```python
from build123d import *

# Parameters (mm, degrees)
P_IDAT_VYSUNUT_M1_DEPTH  = 8
SKICA2_R                 = 2.2
ODEBRAT_VYSUNUT_M1_DEPTH = 8
P_IDAT_VYSUNUT_M3_DEPTH  = 15
ZAOBLIT3_R               = 10
ZAOBLIT5_R               = 2
ZAOBLIT6_R               = 2
ZAOBLIT7_R               = 2
P_IDAT_VYSUNUT_M6_DEPTH  = 23
ZAOBLIT12_R              = 2
ZAOBLIT13_R              = 2
ZAOBLIT14_R              = 2
ZAOBLIT15_R              = 2
ODEBRAT_VYSUNUT_M4_DEPTH = 8.5
ZAOBLIT18_R              = 2
ZAOBLIT19_R              = 2
SKICA8_R                 = 0.5000000000000009
SKICA8_W                 = 12.000000000000004
SKICA8_H                 = 9
ODEBRAT_VYSUNUT_M5_DEPTH = 2
SKICA9_W                 = 12.000000000000004
SKICA9_H                 = 9
ODEBRAT_VYSUNUT_M6_DEPTH = 2.5


with BuildPart() as part:
    # Skica1 → Přidat vysunutím1 (new body)
    with BuildSketch(Plane.XY):
        Polygon((0, 0), (0, 25), (35, 25.000000000000004), (35, -3.47e-15), align=None)
        Polygon((3.999999999999999, 18.500000000000004), (4, 6.500000000000001), (18, 6.500000000000001), (20.485281374238575, 12.499999999999996), (18, 18.499999999999996), align=None, mode=Mode.SUBTRACT)
    extrude(amount=P_IDAT_VYSUNUT_M1_DEPTH)

    # Skica2 → Odebrat vysunutím1 (cut)
    with BuildSketch(Plane.ZY):
        with Locations((4, 12.5)):
            Circle(SKICA2_R)
    extrude(amount=-ODEBRAT_VYSUNUT_M1_DEPTH, mode=Mode.SUBTRACT)

    # Skica3 → Přidat vysunutím3 (add)
    with BuildSketch(Plane(origin=(0, 0, 0), x_dir=(-1, 0, 0), z_dir=(0, 0, -1))):
        Polygon((-35, 25.000000000000004), (-22, 25.000000000000004), (-21.999999999999996, 0), (-35, 0), align=None)
    extrude(amount=P_IDAT_VYSUNUT_M3_DEPTH)

    # Zaoblit3
    # the kernel refuses this fillet: 10 mm, written as the material it adds along each edge
    with BuildSketch(Plane(origin=(22, 25.000000000000004, 0), x_dir=(0, 0, -1), z_dir=(-1.4e-16, -1, 0))) as zaoblit3_piece_1_section:
        with BuildLine():
            CenterArc((ZAOBLIT3_R, -ZAOBLIT3_R), ZAOBLIT3_R, 90, 90)
            Line((-1.78e-15, -ZAOBLIT3_R), (0, 0))
            Line((0, 0), (ZAOBLIT3_R, 0))
        make_face()
    zaoblit3_piece_1 = extrude(amount=49.99999999999999, mode=Mode.PRIVATE)
    zaoblit3_piece_1 = split(zaoblit3_piece_1, bisect_by=Plane(origin=(17.13517134220591, 20.587881074775396, -2.4104777479798574), z_dir=(0.9238795325112865, 0.3826834323650904, 0)), keep=Keep.TOP, mode=Mode.PRIVATE)
    add(zaoblit3_piece_1)
    with BuildSketch(Plane(origin=(22, 25.000000000000004, 0), x_dir=(0, 0, -1), z_dir=(-1.4e-16, -1, 0))) as zaoblit3_piece_2_section:
        with BuildLine():
            CenterArc((ZAOBLIT3_R, -ZAOBLIT3_R), ZAOBLIT3_R, 90, 90)
            Line((-1.78e-15, -ZAOBLIT3_R), (0, 0))
            Line((0, 0), (ZAOBLIT3_R, 0))
        make_face()
    zaoblit3_piece_2 = extrude(amount=49.99999999999999, mode=Mode.PRIVATE)
    zaoblit3_piece_2 = split(zaoblit3_piece_2, bisect_by=Plane(origin=(15.789776111016284, 18.499999999999996, -0.41218867261979963), z_dir=(5.1e-16, 1, 0)), keep=Keep.TOP, mode=Mode.PRIVATE)
    add(zaoblit3_piece_2)
    with BuildSketch(Plane(origin=(22.000000000000004, 50, 0), x_dir=(0, 0, -1), z_dir=(-1.4e-16, -1, 0))) as zaoblit3_piece_3_section:
        with BuildLine():
            CenterArc((ZAOBLIT3_R, -ZAOBLIT3_R), ZAOBLIT3_R, 90, 90)
            Line((-1.78e-15, -ZAOBLIT3_R), (0, 0))
            Line((0, 0), (ZAOBLIT3_R, 0))
        make_face()
    zaoblit3_piece_3 = extrude(amount=50, mode=Mode.PRIVATE)
    zaoblit3_piece_3 = split(zaoblit3_piece_3, bisect_by=Plane(origin=(15.78977611101612, 6.500000000000001, -0.41218867261958336), z_dir=(0, -1, 0)), keep=Keep.TOP, mode=Mode.PRIVATE)
    add(zaoblit3_piece_3)
    with BuildSketch(Plane(origin=(22.000000000000004, 50, 0), x_dir=(0, 0, -1), z_dir=(-1.4e-16, -1, 0))) as zaoblit3_piece_4_section:
        with BuildLine():
            CenterArc((ZAOBLIT3_R, -ZAOBLIT3_R), ZAOBLIT3_R, 90, 90)
            Line((-1.78e-15, -ZAOBLIT3_R), (0, 0))
            Line((0, 0), (ZAOBLIT3_R, 0))
        make_face()
    zaoblit3_piece_4 = extrude(amount=50, mode=Mode.PRIVATE)
    zaoblit3_piece_4 = split(zaoblit3_piece_4, bisect_by=Plane(origin=(19.135383660262896, 9.241058631103481, -2.632109872171155), z_dir=(0.9238795325112864, -0.38268343236509067, 0)), keep=Keep.TOP, mode=Mode.PRIVATE)
    add(zaoblit3_piece_4)

    # Zaoblit5
    # the kernel refuses this fillet: 2 mm, written as the material it takes off along each edge
    with BuildSketch(Plane(origin=(0, -5, 0), x_dir=(0, 0, 1), z_dir=(0, 1, 0))) as zaoblit5_piece_1:
        with BuildLine():
            CenterArc((ZAOBLIT5_R, ZAOBLIT5_R), ZAOBLIT5_R, 180, 90)
            Line((-2.2e-16, ZAOBLIT5_R), (0, 0))
            Line((0, 0), (ZAOBLIT5_R, 0))
        make_face()
    extrude(amount=35, mode=Mode.SUBTRACT)

    # Zaoblit6
    zaoblit6_edges = [part.edges().sort_by_distance(p)[0] for p in [
        (21.999999999999996, 0, -12.5),
        (19.071067811865476, 0, -2.9289321881345254),
        (7, -6.9e-16, 0),
        (0.5857864376269049, 0, 0.5857864376269051),
        (0, 0, 5),
    ]]
    fillet(zaoblit6_edges, radius=ZAOBLIT6_R)

    # Zaoblit7
    zaoblit7_edges = [part.edges().sort_by_distance(p)[0] for p in [
        (22, 25.000000000000004, -12.5),
        (7, 25, 0),
        (19.071067811865476, 25, -2.9289321881345245),
        (0.5857864376269049, 25, 0.5857864376269051),
        (0, 25, 5),
    ]]
    fillet(zaoblit7_edges, radius=ZAOBLIT7_R)

    # Skica6 → Přidat vysunutím6 (add)
    with BuildSketch(Plane(origin=(0, 0, -15), x_dir=(-1, 0, 0), z_dir=(0, 0, -1))):
        with BuildLine():
            Line((-35, 23.500000000000004), (-35, 1.5))
            ThreePointArc((-35, 1.5), (-35.60000000229765, 2.1000000000000085), (-36.2, 1.4999999954047263))
            ThreePointArc((-36.2, 1.4999999954047263), (-36.58, 1.1199999924943909), (-36.96, 1.4999999954047263))
            Line((-36.96, 1.4999999954047263), (-36.959999999999994, 23.500000000000096))
            ThreePointArc((-36.959999999999994, 23.500000000000096), (-36.58, 23.88000000000009), (-36.2, 23.500000000000096))
            ThreePointArc((-36.2, 23.500000000000096), (-35.60000000000006, 22.9), (-35, 23.500000000000004))
        make_face()
    extrude(amount=-P_IDAT_VYSUNUT_M6_DEPTH)

    # Zaoblit12
    zaoblit12_edges = [part.edges().sort_by_distance(p)[0] for p in [
        (29.5, 0, -15),
        (22.5857864376269, 0.5857864376269046, -15),
        (29.5, 25.000000000000004, -15),
        (22.585786437626904, 24.414213562373096, -15),
        (21.999999999999996, 12.5, -15),
    ]]
    fillet(zaoblit12_edges, radius=ZAOBLIT12_R)

    # Zaoblit13
    zaoblit13_edges = [part.edges().sort_by_distance(p)[0] for p in [
        (20.485281374238724, 12.499999999999886, 1.6457513110643447),
    ]]
    fillet(zaoblit13_edges, radius=ZAOBLIT13_R)

    # Zaoblit14
    zaoblit14_edges = [part.edges().sort_by_distance(p)[0] for p in [
        (17.99999999999998, 18.500000000000004, 3.000000000000016),
    ]]
    fillet(zaoblit14_edges, radius=ZAOBLIT14_R)

    # Zaoblit15
    zaoblit15_edges = [part.edges().sort_by_distance(p)[0] for p in [
        (18.0000000000001, 6.499999999999996, 2.9999999999999263),
    ]]
    fillet(zaoblit15_edges, radius=ZAOBLIT15_R)

    # Skica7 → Odebrat vysunutím4 (cut)
    with BuildSketch(Plane(origin=(36.96, 1.166e-14, 0), x_dir=(0, 0, -1), z_dir=(1, 0, 0))):
        Polygon((-8, 21.00000000000012), (15, 21.00000000000012), (15.000000000000005, 4.000000000000118), (-7.999999999999998, 4.000000000000118), align=None)
    extrude(amount=-ODEBRAT_VYSUNUT_M4_DEPTH, mode=Mode.SUBTRACT)

    # Zaoblit18
    zaoblit18_edges = [part.edges().sort_by_distance(p)[0] for p in [
        (36.96, 21.00000000000013, -3.5),
    ]]
    fillet(zaoblit18_edges, radius=ZAOBLIT18_R)

    # Zaoblit19
    zaoblit19_edges = [part.edges().sort_by_distance(p)[0] for p in [
        (36.96, 4.00000000000013, -3.5000000000000036),
    ]]
    fillet(zaoblit19_edges, radius=ZAOBLIT19_R)

    # Skica8 → Odebrat vysunutím5 (cut)
    with BuildSketch(Plane(origin=(28.46, 0, 0), x_dir=(0, 0, -1), z_dir=(1, 0, 0))):
        with Locations((-4.750000000000001, 18.50000000000013)):
            Circle(SKICA8_R)
        with Locations((-4.750000000000001, 6.500000000000129)):
            Circle(SKICA8_R)
        with Locations((10.750000000000002, 18.50000000000013)):
            Circle(SKICA8_R)
        with Locations((10.750000000000002, 6.500000000000129)):
            Circle(SKICA8_R)
        with Locations((3.000000000000002, 12.500000000000128)):
            Rectangle(SKICA8_W, SKICA8_H)
    extrude(amount=-ODEBRAT_VYSUNUT_M5_DEPTH, mode=Mode.SUBTRACT)

    # Skica9 → Odebrat vysunutím6 (cut)
    with BuildSketch(Plane(origin=(28.46, 0, 0), x_dir=(0, 0, -1), z_dir=(1, 0, 0))):
        Polygon((-3.250000000000001, 17.000000000000128), (-5.999999999999998, 17.000000000000128), (-5.999999999999997, 8.000000000000128), (-3.2500000000000004, 8.000000000000128), (-2.9999999999999987, 8.000000000000128), (-2.9999999999999987, 17.000000000000128), align=None)
        Polygon((-3.250000000000001, 18.50000000000013), (-3.250000000000001, 17.000000000000128), (-2.9999999999999987, 17.000000000000128), (9.000000000000004, 17.000000000000128), (9.250000000000002, 17.000000000000128), (9.250000000000002, 18.50000000000013), align=None)
        Polygon((9.250000000000002, 17.000000000000128), (9.000000000000004, 17.000000000000128), (9.000000000000004, 8.000000000000128), (9.250000000000004, 8.000000000000128), (13.500000000000004, 8.000000000000128), (13.500000000000002, 17.000000000000128), align=None)
        with Locations((3.000000000000002, 12.500000000000128)):
            Rectangle(SKICA9_W, SKICA9_H)
        Polygon((-2.9999999999999987, 8.000000000000128), (-3.2500000000000004, 8.000000000000128), (-3.2500000000000004, 6.500000000000129), (9.250000000000002, 6.500000000000129), (9.250000000000002, 8.000000000000128), (9.000000000000004, 8.000000000000128), align=None)
    extrude(amount=-ODEBRAT_VYSUNUT_M6_DEPTH, mode=Mode.SUBTRACT)


solid = part.part
```
Here's how the part is built. I have some questions about the finished solid (model axes, mm). A direction names the side the tool comes from. Give positions to 0.01 mm unless a question says otherwise; leave off trailing zeros. Loops run counter-clockwise (first coordinate to the right, second up) from the corner with the lowest first, then second, coordinate; pieces in that order, holes last. Notation, with made-up numbers: M 53.25,-34.75 L 73.25,-34.75 A12 ccw 73.25,-20.75 Z; hole C 63,-40 d3. An arc over 180 degrees is marked long. Return JSON: item names as keys, results as strings.
Item 1: Thinking about a two-plate mould opening in X: for faces 1 (the cylindrical face through (21.109, 12.647, -5.874)), 2 (the flat face through (10, 18.5, 3)), 3 (the flat face through (27, 18.5, -3)), 4 (the flat face through (19.33, 9.71, 1.97)), which applies, released by +X, released by -X, zero draft, split by the parting line, or undercut?
A:
{"face 1": "released by -X", "face 2": "undercut", "face 3": "zero draft", "face 4": "undercut"}
Item 2: Imagine slicing it at A-A on x = 8. List the corners of the cut face in (y, z) for me.
A:
{"outline": "M 0,2 A2 ccw 2,0 L 6.5,0 L 6.5,8 L 0,8 Z; M 18.5,0 L 23,0 A2 ccw 25,2 L 25,8 L 18.5,8 Z"}
Item 3: I'm going to push flat-ended pins straight in: pin 1 Ø10 at (y, z) = (18, -0.5) entering from -X; pin 2 Ø6 at (x, y) = (15.5, 4.5) entering from -Z; pin 3 Ø0.9 at (y, z) = (16, -12) entering from -X; pin 4 Ø11 at (x, y) = (7, 11) entering from -Z. Where does each tip first touch, or does it pass through?
A:
{"pin 1": "stops at x = 0", "pin 2": "stops at z = -2.4", "pin 3": "stops at x = 22", "pin 4": "stops at z = 0"}
Item 4: On a 3-axis mill with a long thin cutter (end or side, diameter ignored), from which of +Z, -Z, +X, -X, +Y, -Y can I reach the whole of each face in a straight line? I mean faces 5 (the cylindrical face through (20.32, 12.51, 1.86)), 6 (the flat face through (28.46, 5, -4)), 7 (the flat face through (27, 17, -11)), 8 (the cylindrical face through (29.56, 24.4, -14.43)). Say none if no direction works.
A:
{"face 5": "+Z, -Z", "face 6": "+Z, -Z, +X", "face 7": "+X", "face 8": "-Z, -X, +Y"}
Item 5: Imagine slicing it at D-D on y = 15.25. List the corners of the cut face in (x, z) for me, then the cut area to 3 significant figures.
A:
{"outline": "M 0,2 A2 ccw 2,0 L 4,0 L 4,8 L 0,8 Z; M 19.35,-3.22 A10 cw 22,-10 L 22,-13 A2 ccw 24,-15 L 28.46,-15 L 28.46,-13.5 L 25.96,-13.5 L 25.96,6 L 28.46,6 L 28.46,8 L 19.35,8 Z", "area": "166 mm^2"}
Item 6: Imagine slicing it at C-C on y = 5. List the corners of the cut face in (x, z) for me, then the cut area to 3 significant figures.
A:
{"outline": "M 0,2 A2 ccw 2,0 L 12,0 A10 cw 22,-10 L 22,-13 A2 ccw 24,-15 L 28.46,-15 L 28.46,8 L 0,8 Z", "area": "344 mm^2"}
Item 7: Please list where these lines run through material, in increasing order: line 1 (Y direction, x = 27.3, z = -10.75); line 2 (Z direction, x = 27.5, y = 13.25); line 3 (Y direction, x = 2.3, z = 4).
A:
{"line 1": "y = 0 to 6, 7 to 8, 17 to 18, 19 to 25", "line 2": "z = -15 to -13.5, 6 to 8", "line 3": "y = 0 to 10.3, 14.7 to 25"}
